Check sheet for the modelled part. Datum: model origin and axes. Units: mm. A direction names the side the tool comes from. Round coordinates to 2 decimals unless told otherwise and drop trailing zeros. Loops run counter-clockwise (first coordinate to the right, second up) from the corner with the lowest first, then second, coordinate; pieces in that order, holes last. Notation, with made-up numbers: (6.5, 33.25) - (65.5, 33.25) arc R26 ccw to (65.5, 50.25) - close; hole circle Ø8 at (18.5, 81.25). An arc over 180 degrees is marked (long way). Put each result on its own line as item: value.
```python
from build123d import *

# Parameters (mm, degrees)
SKETCH1_W                = 25
SKETCH1_H                = 25
BOSS_EXTRUDE1_DEPTH      = 2
BOSS_EXTRUDE2_DEPTH      = 15
BOSS_EXTRUDE2_DEPTH_BACK = 2
SKETCH2_W                = 25
SKETCH2_H                = 2
SKETCH3_R                = 2.025
CUT_EXTRUDE1_DEPTH       = 35.960692213
FILLET1_R                = 2
FILLET2_R                = 1
SKETCH4_W                = 21
SKETCH4_H                = 2
BOSS_EXTRUDE3_DEPTH      = 3
SKETCH5_W                = 21
SKETCH5_H                = 2
BOSS_EXTRUDE4_DEPTH      = 15
BOSS_EXTRUDE5_DEPTH      = 15
BOSS_EXTRUDE5_DEPTH_BACK = 36
SKETCH6_W                = 10
SKETCH6_H                = 2
SKETCH7_W                = 2
SKETCH7_H                = 41
BOSS_EXTRUDE6_DEPTH      = 105
SKETCH8_W                = 10
SKETCH8_H                = 4
CUT_EXTRUDE2_DEPTH       = 118.389309564
FILLET3_R                = 1
FILLET4_R                = 2
SKETCH12_R               = 7.025
CUT_EXTRUDE4_DEPTH       = 119.102709537
CUT_EXTRUDE5_DEPTH       = 119.102709537
FILLET7_R                = 6
FILLET8_R                = 6
SKETCH14_W               = 10
SKETCH14_H               = 5
CUT_EXTRUDE6_DEPTH       = 112.496636721
SKETCH15_W               = 15
SKETCH15_H               = 54
CUT_EXTRUDE7_DEPTH       = 117.405541105
SKETCH16_W               = 10
SKETCH16_H               = 8
CUT_EXTRUDE8_DEPTH       = 10


with BuildPart() as part:
    # Sketch1 → Boss-Extrude1 (new body)
    with BuildSketch(Plane(origin=(0, 0, 0), x_dir=(1, 0, 0), z_dir=(0, 1, 0))):
        Rectangle(SKETCH1_W, SKETCH1_H)
    extrude(amount=BOSS_EXTRUDE1_DEPTH)

    # Sketch2 → Boss-Extrude2 (add, two sides: drawn at the far end of the back side and taken through both)
    with BuildSketch(Plane.XZ.offset(-BOSS_EXTRUDE2_DEPTH_BACK)):
        with Locations((0, 13.5)):
            Rectangle(SKETCH2_W, SKETCH2_H)
        with Locations((0, -13.5)):
            Rectangle(SKETCH2_W, SKETCH2_H)
    extrude(amount=BOSS_EXTRUDE2_DEPTH + BOSS_EXTRUDE2_DEPTH_BACK)

    # Sketch3 → Cut-Extrude1 (cut, through all)
    with BuildSketch(Plane.XY.offset(14.5)):
        with Locations((-9.5, -10)):
            Circle(SKETCH3_R)
        with Locations((5.5, -10)):
            Circle(SKETCH3_R)
    extrude(amount=-CUT_EXTRUDE1_DEPTH, mode=Mode.SUBTRACT)

    # Fillet1
    fillet1_edges = [part.edges().sort_by_distance(p)[0] for p in [
        (0, 2, 14.5),
        (0, 2, -14.5),
    ]]
    fillet(fillet1_edges, radius=FILLET1_R)

    # Fillet2
    fillet2_edges = [part.edges().sort_by_distance(p)[0] for p in [
        (0, 0, 12.5),
        (0, 0, -12.5),
    ]]
    fillet(fillet2_edges, radius=FILLET2_R)

    # Sketch4 → Boss-Extrude3 (add)
    with BuildSketch(Plane.ZY.offset(12.5)):
        with Locations((0, 1)):
            Rectangle(SKETCH4_W, SKETCH4_H)
    extrude(amount=BOSS_EXTRUDE3_DEPTH)

    # Sketch5 → Boss-Extrude4 (add)
    with BuildSketch(Plane(origin=(12.5, 0, 0), x_dir=(0, 0, -1), z_dir=(1, 0, 0))):
        with Locations((0, 1)):
            Rectangle(SKETCH5_W, SKETCH5_H)
    extrude(amount=BOSS_EXTRUDE4_DEPTH)

    # Sketch6 → Boss-Extrude5 (add, two sides: drawn at the far end of the back side and taken through both)
    with BuildSketch(Plane.XY.offset(10.5).offset(-BOSS_EXTRUDE5_DEPTH_BACK)):
        with Locations((22.5, 1)):
            Rectangle(SKETCH6_W, SKETCH6_H)
    extrude(amount=BOSS_EXTRUDE5_DEPTH + BOSS_EXTRUDE5_DEPTH_BACK)

    # Sketch7 → Boss-Extrude6 (add)
    with BuildSketch(Plane(origin=(0, 2, 0), x_dir=(1, 0, 0), z_dir=(0, 1, 0))):
        with Locations((-14.5, 0)):
            Rectangle(SKETCH7_W, SKETCH7_H)
    extrude(amount=BOSS_EXTRUDE6_DEPTH)

    # Sketch8 → Cut-Extrude2 (cut, through all)
    with BuildSketch(Plane(origin=(-13.5, 0, 0), x_dir=(0, 0, -1), z_dir=(1, 0, 0))):
        with Locations((-15.5, 4)):
            Rectangle(SKETCH8_W, SKETCH8_H)
        with Locations((15.5, 4)):
            Rectangle(SKETCH8_W, SKETCH8_H)
    extrude(amount=-CUT_EXTRUDE2_DEPTH, mode=Mode.SUBTRACT)

    # Fillet3
    fillet3_edges = [part.edges().sort_by_distance(p)[0] for p in [
        (-13.5, 2, 0),
    ]]
    fillet(fillet3_edges, radius=FILLET3_R)

    # Fillet4
    fillet4_edges = [part.edges().sort_by_distance(p)[0] for p in [
        (-15.5, 0, 0),
    ]]
    fillet(fillet4_edges, radius=FILLET4_R)

    # Sketch12 → Cut-Extrude4 (cut, through all)
    with BuildSketch(Plane.ZY.offset(15.5)):
        with Locations((0, 97)):
            Circle(SKETCH12_R)
    extrude(amount=-CUT_EXTRUDE4_DEPTH, mode=Mode.SUBTRACT)

    # Sketch13 → Cut-Extrude5 (cut, through all)
    with BuildSketch(Plane.ZY.offset(15.5)):
        Polygon((-20.5, 107), (-20.5, 52), (-12.5, 60), (-12.5, 107), align=None)
        Polygon((12.5, 60), (12.5, 107), (20.5, 107), (20.5, 52), align=None)
    extrude(amount=-CUT_EXTRUDE5_DEPTH, mode=Mode.SUBTRACT)

    # Fillet7
    fillet7_edges = [part.edges().sort_by_distance(p)[0] for p in [
        (-14.5, 107, 12.5),
        (-14.5, 107, -12.5),
    ]]
    fillet(fillet7_edges, radius=FILLET7_R)

    # Fillet8
    fillet8_edges = [part.edges().sort_by_distance(p)[0] for p in [
        (-14.5, 6, 20.5),
        (-14.5, 6, -20.5),
    ]]
    fillet(fillet8_edges, radius=FILLET8_R)

    # Sketch14 → Cut-Extrude6 (cut, through all)
    with BuildSketch(Plane(origin=(0, 2, 0), x_dir=(1, 0, 0), z_dir=(0, 1, 0))):
        with Locations((22.5, 23)):
            Rectangle(SKETCH14_W, SKETCH14_H)
        with Locations((22.5, -23)):
            Rectangle(SKETCH14_W, SKETCH14_H)
    extrude(amount=-CUT_EXTRUDE6_DEPTH, mode=Mode.SUBTRACT)

    # Sketch15 → Cut-Extrude7 (cut, through all)
    with BuildSketch(Plane(origin=(-13.5, 0, 0), x_dir=(0, 0, -1), z_dir=(1, 0, 0))):
        with Locations((-20, 33)):
            Rectangle(SKETCH15_W, SKETCH15_H)
        with Locations((20, 33)):
            Rectangle(SKETCH15_W, SKETCH15_H)
    extrude(amount=-CUT_EXTRUDE7_DEPTH, mode=Mode.SUBTRACT)

    # Sketch16 → Cut-Extrude8 (cut)
    with BuildSketch(Plane(origin=(0, 2, 0), x_dir=(1, 0, 0), z_dir=(0, 1, 0))):
        with Locations((22.5, -16.5)):
            Rectangle(SKETCH16_W, SKETCH16_H)
        with Locations((22.5, 16.5)):
            Rectangle(SKETCH16_W, SKETCH16_H)
    extrude(amount=-CUT_EXTRUDE8_DEPTH, mode=Mode.SUBTRACT)


solid = part.part
```
Item 1: Section check C-C on x = 5.5. Enter the section's corners in (y, z) (3 decimals).
Filled sheet:
outline: (-15, -14.5) - (-12.025, -14.5) - (-12.025, -12.5) - (-15, -12.5) - close; (-15, 12.5) - (-12.025, 12.5) - (-12.025, 14.5) - (-15, 14.5) - close; (-7.975, -14.5) - (0, -14.5) arc R2 ccw to (2, -12.5) - (2, 12.5) arc R2 ccw to (0, 14.5) - (-7.975, 14.5) - (-7.975, 12.5) - (-1, 12.5) arc R1 cw to (0, 11.5) - (0, -11.5) arc R1 cw to (-1, -12.5) - (-7.975, -12.5) - close
Item 2: Release check for a two-part mould opening along Y. For faces 1 (the cylindrical face through (-9.939, -11.977, 13.514)), 2 (the flat face through (7, 0, 0)), 3 (the flat face through (7, 2, 0)), 4 (the flat face through (0, -7, 14.5)) record: +Y half, -Y half, draft (parallel to the pull), parting line (faces both ways), or undercut.
Filled sheet:
face 1: undercut
face 2: -Y half
face 3: +Y half
face 4: draft
Item 3: Section check D-D on y = 97. Enter the section's corners in (x, z) (3 decimals).
Filled sheet:
outline: (-15.5, -12.5) - (-13.5, -12.5) - (-13.5, -7.025) - (-15.5, -7.025) - close; (-15.5, 7.025) - (-13.5, 7.025) - (-13.5, 12.5) - (-15.5, 12.5) - close
Item 4: Tool access check on faces 5 (the flat face through (-14, 3, 10.5)), 6 (the flat face through (17.5, 1, -12)), 7 (the flat face through (-12.5, -6, 13)), 8 (the flat face through (22, 1, 12.5)), 9 (the flat face through (-13.5, 54, 0)). Record the directions out of +Z, -Z, +X, -X, +Y, -Y that give a thin tool (end or side, any length) a straight path to the whole face; none if there is none.
Filled sheet:
face 5: +Z, -X, -Y
face 6: -Z, +Y, -Y
face 7: +Z, -X, +Y, -Y
face 8: +Z, +X, +Y, -Y
face 9: +Z, -Z, +X, +Y
Item 5: Go/stop test with flat-tipped pins: pin 1 (1 mm diameter, centred on x = 7, z = 9.5, fed in from -Y); pin 2 (2 mm diameter, centred on x = 14, y = 1, fed in from -Z); pin 3 (0.9 mm diameter, centred on x = -14, y = 4.5, fed in from +Z). Record where each tip stops, or that it passes through.
Filled sheet:
pin 1: y = 0
pin 2: z = -10.5
pin 3: z = 10.5
Item 6: Thickness scan on line 1 (Y direction, x = -1.5, z = 5.75); line 2 (Y direction, x = -9.5, z = 13.85) (3 decimals); line 3 (Y direction, x = -9.5, z = -13.3) (3 decimals). Record the ranges inside material, lowest first. Write a range as from..to.
Filled sheet:
line 1: 0..2
line 2: -15..-12.025, -7.975..1.476
line 3: -15..-12.025, -7.975..1.833
Item 7: Section check B-B on z = 0. Enter the section's corners in (x, y) (3 decimals), then the cut area to 3 significant figures.
Filled sheet:
outline: (-15.5, 2) arc R2 ccw to (-13.5, 0) - (27.5, 0) - (27.5, 2) - (-12.5, 2) arc R1 cw to (-13.5, 3) - (-13.5, 89.975) - (-15.5, 89.975) - close; (-15.5, 104.025) - (-13.5, 104.025) - (-13.5, 107) - (-15.5, 107) - close
area: 267 mm²
Item 8: Section check A-A on y = -6. Enter the section's corners in (x, z), then the cut area to 3 significant figures.
Filled sheet:
outline: (-12.5, -14.5) - (12.5, -14.5) - (12.5, -12.5) - (-12.5, -12.5) - close; (-12.5, 12.5) - (12.5, 12.5) - (12.5, 14.5) - (-12.5, 14.5) - close
area: 100 mm²
